```python
from build123d import *

# Parameters (mm, degrees)
ESBO_O1_R                = 2.5
ESBO_O1_R_2              = 2.499999997
ESBO_O1_R_3              = 2.500000003
RESSALTO_EXTRUS_O1_DEPTH = 3


with BuildPart() as part:
    # Esboço1 → Ressalto-extrusão1 (new body)
    with BuildSketch(Plane(origin=(0, 0, 0), x_dir=(1, 0, 0), z_dir=(0, 1, 0))):
        Polygon((-57.924923454, 7.893845864), (-54.924923454, 7.893845864), (-54.924923454, 10.893845864), (26.768392501, 10.893845864), (26.768392501, 7.893845864), (29.768392501, 7.893845864), (29.768392501, 3.093845864), (26.770408679, 3.093845864), (26.770408679, -1.706154136), (29.770408679, -1.706154136), (29.770408679, -6.506154136), (26.770408679, -6.506154136), (26.770408679, -11.306154136), (29.770408679, -11.306154136), (29.770408679, -16.105925898), (26.770408679, -16.105925898), (26.770408679, -19.105925898), (-55.029591321, -19.105925898), (-55.029591321, -16.105925898), (-58.029591321, -16.105925898), (-58.029591321, -11.306154136), (-54.931224008, -11.306154136), (-54.931224008, -6.506154136), (-57.931224008, -6.506154136), (-57.931224008, -1.706154136), (-54.934182698, -1.706154136), (-54.934182698, 3.093845864), (-57.924923454, 3.093845864), align=None)
        with Locations(Location((-16.621271344, -4.105925898, 0), (0, 0, 270))):
            Circle(ESBO_O1_R, mode=Mode.SUBTRACT)
        with Locations(Location((-16.621271344, 2.144074102, 0), (0, 0, 270))):
            Circle(ESBO_O1_R, mode=Mode.SUBTRACT)
        with Locations(Location((-4.121271344, -4.105925898, 0), (0, 0, 270))):
            Circle(ESBO_O1_R_2, mode=Mode.SUBTRACT)
        with Locations(Location((-16.621271344, -10.355925898, 0), (0, 0, 270))):
            Circle(ESBO_O1_R, mode=Mode.SUBTRACT)
        with Locations(Location((-29.121271344, -4.105925898, 0), (0, 0, 270))):
            Circle(ESBO_O1_R_3, mode=Mode.SUBTRACT)
    extrude(amount=RESSALTO_EXTRUS_O1_DEPTH)


solid = part.part
```
The model under review builds one solid part; all positions refer to its coordinate system, in mm. A direction names the side the tool comes from. Give positions to 0.01 mm unless a question says otherwise; leave off trailing zeros. Loops run counter-clockwise (first coordinate to the right, second up) from the corner with the lowest first, then second, coordinate; pieces in that order, holes last. Notation, with made-up numbers: (-30, -26) -> (-20, -26) arc R33 ccw to (-20, 13) -> close; hole circle Ø2 at (-21.5, 43.25). An arc over 180 degrees is marked (long way). Use CSV: the item, a comma, the result in double quotes.
1. Consider section C-C, the plane z = 9.25. Write out the cut boundary in (x, y).
Result:
outline,"(-54.93, 0) -> (-18.86, 0) -> (-18.86, 3) -> (-54.93, 3) -> close; (-14.38, 0) -> (26.77, 0) -> (26.77, 3) -> (-14.38, 3) -> close"
2. Consider section D-D, the plane z = 17. Write out the cut boundary in (x, y).
Result:
outline,"(-55.03, 0) -> (26.77, 0) -> (26.77, 3) -> (-55.03, 3) -> close"
3. Consider section B-B, the plane y = 1.5. Count the separate pieces of the cut face and the enclosed holes in it, then the cut area to 3 significant figures.
Result:
separate pieces,"1"
enclosed holes,"5"
area,"2,440 mm²"
4. For P1, Ø3, axis at x = -4.12, z = 4.11, coming from the -Y side; P2, Ø0.9, axis at y = 2, z = -9, coming from the -X side; P3, Ø8, axis at x = -49, z = 11, coming from the -Y side; P4, Ø0.9, axis at y = 2, z = -0.5, coming from the +X side, all flat-tipped, find the tip position at first contact; note any pin that passes through.
Result:
P1,"passes through"
P2,"stops at x = -54.92"
P3,"stops at y = 0"
P4,"stops at x = 26.77"
5. Machinability: for faces 4 (the face through (28, 1, 16.106)), 5 (the face through (26.768, 1, -9)), 6 (the face through (26.77, 1, 9)), which of the approach directions +Z, -Z, +X, -X, +Y, -Y give a long, thin tool a straight path to every point of the face, cutting with its end or side? Answer none if there is none.
Result:
face 4,"+Z, +X, +Y, -Y"
face 5,"-Z, +X, +Y, -Y"
face 6,"+X, +Y, -Y"
6. To check wall thickness, follow probe 1 along X at (y, z) = (0.9, 3.5); probe 2 along X at (y, z) = (1.35, 0.5); probe 3 along Z at (x, y) = (-29, 1.2). State the ranges of each line that lie inside material, in increasing order. Write a range as from..to.
Result:
probe 1,"x = -57.93..-31.55, -26.7..-19.05, -14.2..-6.55, -1.7..29.77"
probe 2,"x = -54.93..26.77"
probe 3,"z = -10.89..1.61, 6.6..19.11"
7. The part is to be moulded in two halves that separate along Z. For faces 1 (the face through (29.77, 1, 14)), 2 (the face through (-57, 1, 16.106)), 3 (the face through (28, 1, 6.506)), say which applies: +Z half, -Z half, draft (parallel to the pull), parting line (faces both ways), or undercut.
Result:
face 1,"draft"
face 2,"+Z half"
face 3,"undercut"
8. Consider section A-A, the plane z = 3.75. Write out the cut boundary in (x, y).
Result:
outline,"(-57.93, 0) -> (-31.6, 0) -> (-31.6, 3) -> (-57.93, 3) -> close; (-26.65, 0) -> (-19.1, 0) -> (-19.1, 3) -> (-26.65, 3) -> close; (-14.15, 0) -> (-6.6, 0) -> (-6.6, 3) -> (-14.15, 3) -> close; (-1.65, 0) -> (29.77, 0) -> (29.77, 3) -> (-1.65, 3) -> close"
